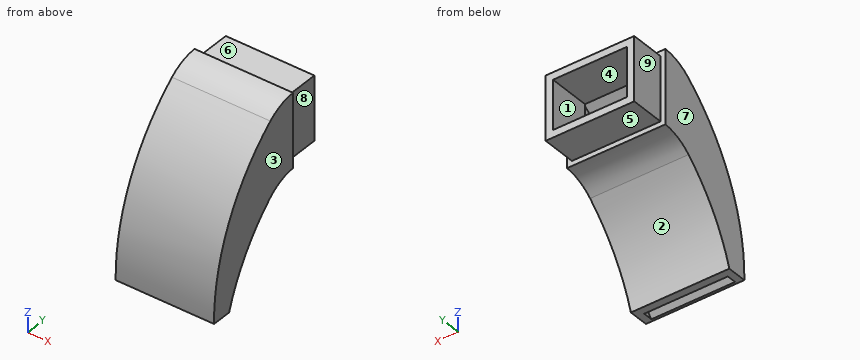
Autodesk Inventor part; units mm, degrees
ref_plane "YZ Plane" through (0, 0, 0) normal (1, 0, 0) x (0, 1, 0)
ref_plane "XZ Plane" through (0, 0, 0) normal (0, 1, 0) x (-1, 0, 0)
ref_plane "XY Plane" through (0, 0, 0) normal (0, 0, 1) x (1, 0, 0)
sketch "Szkic1" plane through (0, 0, 0) normal (0, 1, 0) x (-1, 0, 0)
  line L0 (9, 6.5) -> (-9, 6.5)
  line L1 (-9, 6.5) -> (-9, -6.5)
  line L2 (-9, -6.5) -> (9, -6.5)
  line L3 (9, -6.5) -> (9, 6.5)
  line L4 (9, 0) -> (0, 0) construction
  line L5 (0, 0) -> (0, -6.5) construction
  dimension "d0" = 13
  dimension "d1" = 18
extrude "Wyciągnięcie proste1" add sketch "Szkic1" along normal blind 7
sketch "Szkic2" plane through (0, 0, 0) normal (0, -1, 0) x (1, 0, 0)
  line L0 (-10, 7.5) -> (10, 7.5)
  line L1 (10, 7.5) -> (10, -7.5)
  line L2 (10, -7.5) -> (-10, -7.5)
  line L3 (-10, -7.5) -> (-10, 7.5)
  line L4 (0, 7.5) -> (0, 0) construction
  line L5 (0, 0) -> (10, 0) construction
  dimension "d4" = 20
  dimension "d5" = 15
extrude "Wyciągnięcie proste2" add sketch "Szkic2" along normal blind 3
sketch "Szkic3" plane through (10, 0, 7.5) normal (1, 0, 0) x (0, 0, -1)
  line L0 (0, 0) -> (0, -3)
  arc A0 (0, -3) -> (34, -21) centre (33.4095, 18.9956) ccw
  line L1 (1, 7) -> (14, 7)
  line L2 (0, -3) -> (15, -3)
  arc A1 (15, -3) -> (34, -17) centre (45.9271, 19.0797) ccw
  line L3 (34, -17) -> (34, -21)
  line L4 (15, 0) -> (15, -3)
  line L5 (0, -3) -> (15, -3)
  point P0 (7.5, 0)
  dimension "d10" = 34
  dimension "d11" = 40
  dimension "d12" = 28
  dimension "d13" = 4
  dimension "d14" = 38
extrude "Wyciągnięcie proste3" add sketch "Szkic3" against normal up to surface (20 mm away)
shell "Skorupa1" thickness 1.5 removed faces 2 at (-3, 7, 2.1667) at (-3.3333, -19.6667, -26.5)
fillet "Zaokrąglenie1" radius 10 2 edges at (0, -3, -7.5) (0, -3, 7.5)
chamfer "Faza1" distance 1 angle 45 1 edges at (0, -19.4998, -26.5)
properties part number "45_dysza chłodząca"
Source: CAD feature listing. Evaluate the final solid. Frame: model axes, mm. Face numbers are marked on the shaded views. A direction names the side the tool comes from. Round coordinates to 2 decimals unless told otherwise and drop trailing zeros. Loops run counter-clockwise (first coordinate to the right, second up) from the corner with the lowest first, then second, coordinate; pieces in that order, holes last.
(1) Section query C-C (z = -14). Output: boundary loops of the cut face in (x, y).
From the geometry:
outline: (-10, -19.19) - (10, -19.19) - (10, -10.03) - (-10, -10.03) - close; hole (-8.5, -17.62) - (8.5, -17.62) - (8.5, -11.96) - (-8.5, -11.96) - close
(2) Section query B-B (y = -4.75). Output: boundary loops of the cut face in (x, z).
From the geometry:
outline: (-10, -8.97) - (10, -8.97) - (10, 6.17) - (-10, 6.17) - close; hole (-8.5, -6.92) - (8.5, -6.92) - (8.5, 4.4) - (-8.5, 4.4) - close
(3) Contact query for flat-ended pins moving along their axis: pin 1 Ø2.5 at (x, y) = (2, 2.5) entering from +Z; pin 2 Ø9.5 at (y, z) = (0.5, -2) entering from -X; pin 3 Ø1.5 at (x, y) = (1.5, -6) entering from -Z; pin 4 Ø1.2 at (x, y) = (0.5, -2.5) entering from -Z. Output: stop coordinate, or through.
From the geometry:
pin 1: stops at z = 6.5
pin 2: stops at x = -10
pin 3: stops at z = -10.56
pin 4: stops at z = -8.15
(4) Pull-direction query (X, two-part tool) for the marked faces 1, 2, 3 and 4; classes: +X half, -X half, draft (parallel to the pull), parting line (faces both ways), or undercut.
From the geometry:
face 1: undercut
face 2: draft
face 3: +X half
face 4: undercut
(5) Section query A-A (x = -6). Output: boundary loops of the cut face in (y, z), and give its area (3 significant figures).
From the geometry:
outline: (-21, -26.5) - (-20.5, -26.5) - (-19.5, -25.5) arc R38.5 cw to (-2.55, 6) - (-1.5, 6) - (-1.5, 5) - (7, 5) - (7, 6.5) - (0, 6.5) - (0, 7.5) arc R10 ccw to (-6.02, 5.31) arc R40 ccw to start; (-18.58, -26.5) - (-17, -26.5) arc R38 cw to (-6.15, -10.01) arc R10 cw to (0, -7.5) - (0, -6.5) - (7, -6.5) - (7, -5) - (-1.5, -5) - (-1.5, -6) - (-3.48, -6) arc R39.5 ccw to start
area: 129 mm2
(6) Section query D-D (z = -3). Output: boundary loops of the cut face in (x, y), and give its area (3 significant figures).
From the geometry:
outline: (-10, -13.79) - (10, -13.79) - (10, 0) - (9, 0) - (9, 7) - (7.5, 7) - (7.5, -1.5) - (8.5, -1.5) - (8.5, -11.95) - (-8.5, -11.95) - (-8.5, -1.5) - (-7.5, -1.5) - (-7.5, 7) - (-9, 7) - (-9, 0) - (-10, 0) - close
area: 96.8 mm2
(7) Material intervals for probe 1 along X at (y, z) = (-5, 1); probe 2 along Z at (x, y) = (-1, 5.5); probe 3 along Y at (x, z) = (5.5, -21), sorted ascending.
From the geometry:
probe 1: x = -10 to -8.5, 8.5 to 10
probe 2: z = -6.5 to -5, 5 to 6.5
probe 3: y = -20.7 to -19.19, -16.37 to -14.69
(8) Access query for the marked faces 5, 6, 7, 8 and 9. Directions: +Z, -Z, +X, -X, +Y, -Y. A direction counts if a zero-diameter tool reaches every point of the face in a straight line with its end or side. Return the directions, or none.
From the geometry:
face 5: -Z, +X, -X, +Y
face 6: +Z, +X, -X, +Y
face 7: +Z, -Z, -X, +Y, -Y
face 8: +Z, -Z, +X, +Y
face 9: +Z, -Z, -X, +Y
